For this review, use the dimensioned drawing (mm, ordinates from the lowest corner) and the shaded views. A direction names the side the tool comes from. Coordinates: 2 decimals unless noted, no trailing zeros. Write each loop counter-clockwise with the first axis right and the second up, starting at its lowest first coordinate (ties: lowest second). Pieces come first, ordered by that corner, then holes. Notation, with made-up numbers: M 12.25,52.25 L 19.25,52.25 A21 ccw 19.25,85.25 Z; hole C 32,5 d10. An arc over 180 degrees is marked long. One line per question, with ' | ' between items.
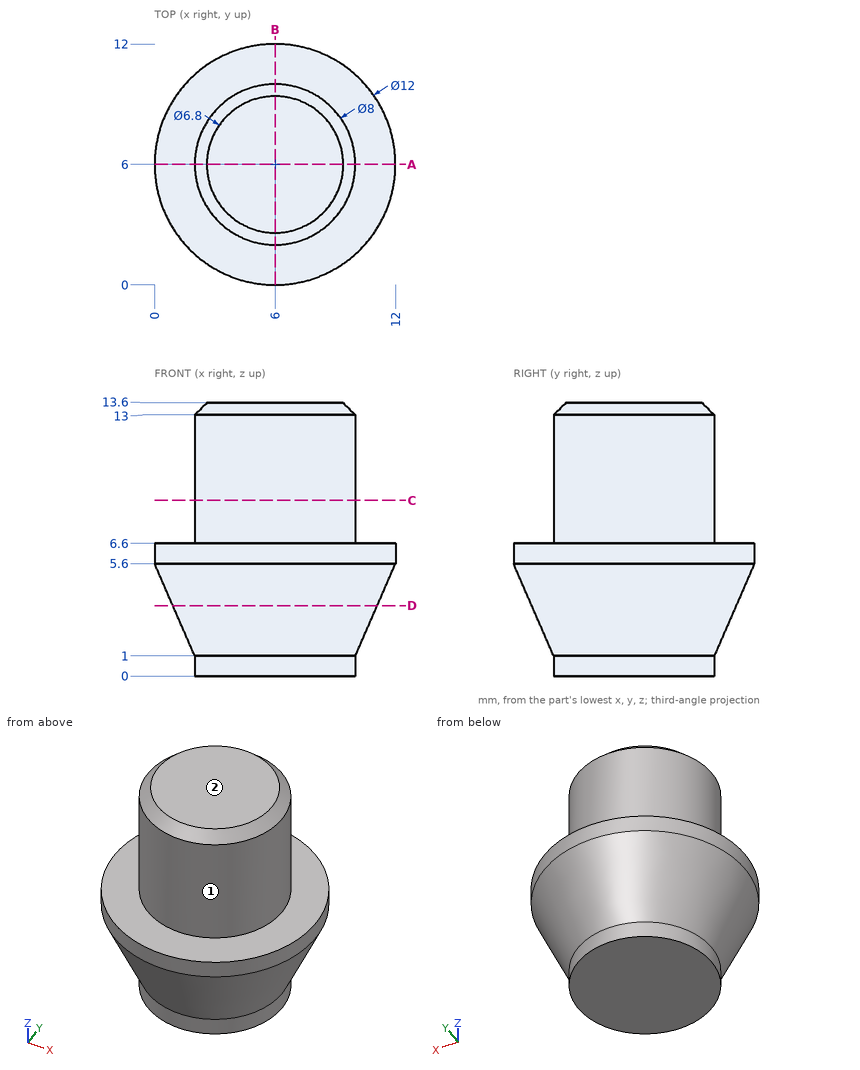
1) Machinability: for the marked faces 1 and 2, which of the approach directions +Z, -Z, +X, -X, +Y, -Y give a long, thin tool a straight path to every point of the face, cutting with its end or side? Answer none if there is none.
Responses:
face 1: +Z | face 2: +Z, +X, -X, +Y, -Y
2) We need section D-D on z = 3.5. State the section outline as (x, y) points, then the cut area to 3 significant figures.
Responses:
outline: C 6,6 d10.17 | area: 81.3 mm^2
3) We need section A-A on y = 6. State the section outline as (x, z) points, then the cut area to 3 significant figures.
Responses:
outline: M 0,5.6 L 2,1 L 2,0 L 10,0 L 10,1 L 12,5.6 L 12,6.6 L 10,6.6 L 10,13 L 9.4,13.6 L 2.6,13.6 L 2,13 L 2,6.6 L 0,6.6 Z | area: 122 mm^2
4) We need section C-C on z = 8.75. State the section outline as (x, y) points, then the cut area to 3 significant figures.
Responses:
outline: C 6,6 d8 | area: 50.3 mm^2
5) To check wall thickness, follow line 1 along X through (y, z) = (3.25, 1.5); line 2 along X through (y, z) = (6, 7.5); line 3 along Z through (x, y) = (10.5, 7.25). State the ranges of each line that lie inside material, in increasing order. Write a range as [from, to].
Responses:
line 1: [2.8, 9.2] | line 2: [2, 10] | line 3: [2.54, 6.6]
6) Insertion check: pin 1 Ø1 at (x, z) = (3, 3.5) entering from +Y; pin 2 Ø3 at (x, z) = (5, 12) entering from -Y; pin 3 Ø6 at (x, z) = (3, 2.5) entering from +Y; pin 4 Ø6 at (y, z) = (7, 3) entering from +X. Each pin has a flat end and moves straight along its axis. Give the tip position at first contact, or say it passes through.
Responses:
pin 1: y = 10.52 | pin 2: y = 2 | pin 3: y = 11.58 | pin 4: x = 12
